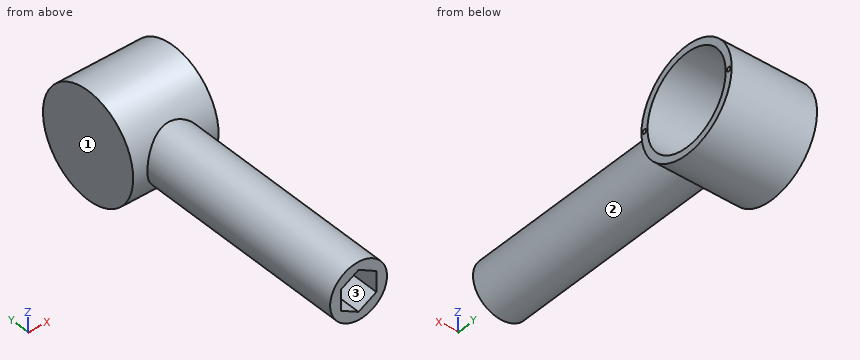
from build123d import *

# Parameters (mm, degrees)
SKETCH1_R                 = 20
BOSS_EXTRUDE1_DEPTH       = 25
BOSS_EXTRUDE2_START       = 100
SKETCH2_R                 = 20
BOSS_EXTRUDE2_DEPTH       = 100
BOSS_EXTRUDE4_START       = -100
SKETCH6_R                 = 20
BOSS_EXTRUDE4_DEPTH       = 100
SKETCH7_R                 = 25
CUT_EXTRUDE2_DEPTH        = 40
SKETCH8_R                 = 25
SKETCH8_R_2               = 22.5
BOSS_EXTRUDE7_DEPTH       = 40
SKETCH9_R                 = 25
BOSS_EXTRUDE8_DEPTH       = 2
BOSS_EXTRUDE10_DEPTH      = 38
CUT_EXTRUDE3_DEPTH        = 25
SKETCH12_R                = 25
CUT_EXTRUDE4_DEPTH        = 75
BOSS_EXTRUDE11_START      = 50
SKETCH14_R                = 20
BOSS_EXTRUDE11_DEPTH      = 50
BOSS_EXTRUDE12_DEPTH      = 10
BOSS_EXTRUDE12_DEPTH_BACK = 50
SKETCH13_R                = 37.5
SKETCH17_R                = 32.5
CUT_EXTRUDE5_DEPTH        = 50
BOSS_EXTRUDE13_START      = 2
SKETCH18_R                = 37.5
SKETCH18_R_2              = 32.5
BOSS_EXTRUDE13_DEPTH      = 2
SKETCH21_R                = 37.5
SKETCH21_R_2              = 32.5
CUT_EXTRUDE6_DEPTH        = 2
SKETCH22_R                = 1.5
CUT_EXTRUDE7_DEPTH        = 10
BOSS_EXTRUDE14_START      = 5
SKETCH27_R                = 32.5
BOSS_EXTRUDE14_DEPTH      = 5


with BuildPart() as part:
    # Sketch1 → Boss-Extrude1 (new body)
    with BuildSketch(Plane(origin=(0, 0, 0), x_dir=(1, 0, 0), z_dir=(0, 1, 0))):
        with Locations(Location((0, 0, 0), (0, 0, 270))):
            Circle(SKETCH1_R)
        Polygon((14.43375673, 0), (7.216878365, 12.5), (-7.216878365, 12.5), (-14.43375673, 0), (-7.216878365, -12.5), (7.216878365, -12.5), align=None, mode=Mode.SUBTRACT)
    extrude(amount=BOSS_EXTRUDE1_DEPTH)

    # Sketch2 → Boss-Extrude2 (add)
    with BuildSketch(Plane.XZ.offset(BOSS_EXTRUDE2_START)):
        with Locations(Location((0, 0, 0), (0, 0, 270))):
            Circle(SKETCH2_R)
    extrude(amount=-BOSS_EXTRUDE2_DEPTH)

    # Sketch6 → Boss-Extrude4 (add)
    with BuildSketch(Plane(origin=(0, 25, 0), x_dir=(1, 0, 0), z_dir=(0, 1, 0)).offset(BOSS_EXTRUDE4_START)):
        with Locations(Location((0, 0, 0), (0, 0, 90))):
            Circle(SKETCH6_R)
    extrude(amount=BOSS_EXTRUDE4_DEPTH)

    # Sketch7 → Cut-Extrude2 (cut)
    with BuildSketch(Plane(origin=(20, 0, 0), x_dir=(0, 0, -1), z_dir=(1, 0, 0))):
        with Locations((0, 39.286563349)):
            Circle(SKETCH7_R)
    extrude(amount=-CUT_EXTRUDE2_DEPTH, mode=Mode.SUBTRACT)

    # Sketch8 → Boss-Extrude7 (add)
    with BuildSketch(Plane(origin=(20, 0, 0), x_dir=(0, 0, -1), z_dir=(1, 0, 0))):
        with Locations((0, 39.252781264)):
            Circle(SKETCH8_R)
        with Locations((0, 39.252781264)):
            Circle(SKETCH8_R_2, mode=Mode.SUBTRACT)
    extrude(amount=-BOSS_EXTRUDE7_DEPTH)

    # Sketch9 → Boss-Extrude8 (add)
    with BuildSketch(Plane(origin=(20, 0, 0), x_dir=(0, 0, -1), z_dir=(1, 0, 0))):
        with Locations((0, 39.252781264)):
            Circle(SKETCH9_R)
    extrude(amount=-BOSS_EXTRUDE8_DEPTH)

    # Sketch10 → Boss-Extrude10 (add)
    with BuildSketch(Plane.ZY.offset(-18)):
        with BuildLine():
            Line((-15.081099266, 22.555163323), (15.081099266, 22.555163323))
            ThreePointArc((15.081099266, 22.555163323), (0, 16.752781264), (-15.081099266, 22.555163323))
        make_face()
    extrude(amount=BOSS_EXTRUDE10_DEPTH)

    # Sketch11 → Cut-Extrude3 (cut)
    with BuildSketch(Plane.XZ.offset(100)):
        Polygon((12.5, 7.216878365), (0, 14.43375673), (0, 0), (12.5, 0), align=None)
        Polygon((0, 0), (0, 14.43375673), (-12.5, 7.216878365), (-12.5, -7.216878365), (0, -14.43375673), (12.5, -7.216878365), (12.5, 0), align=None)
    extrude(amount=-CUT_EXTRUDE3_DEPTH, mode=Mode.SUBTRACT)

    # Sketch12 → Cut-Extrude4 (cut)
    with BuildSketch(Plane(origin=(20, 0, 0), x_dir=(0, 0, -1), z_dir=(1, 0, 0))):
        with Locations((0, 39.252781264)):
            Circle(SKETCH12_R)
    extrude(amount=-CUT_EXTRUDE4_DEPTH, mode=Mode.SUBTRACT)

    # Sketch14 → Boss-Extrude11 (add)
    with BuildSketch(Plane.XZ.offset(100).offset(BOSS_EXTRUDE11_START)):
        with Locations(Location((0, 0, 0), (0, 0, 270))):
            Circle(SKETCH14_R)
        Polygon((0, -14.43375673), (12.5, -7.216878365), (12.5, 7.216878365), (0, 14.43375673), (-12.5, 7.216878365), (-12.5, -7.216878365), align=None, mode=Mode.SUBTRACT)
    extrude(amount=-BOSS_EXTRUDE11_DEPTH)

    # Sketch13 → Boss-Extrude12 (add, two sides: drawn at the far end of the back side and taken through both)
    with BuildSketch(Plane(origin=(20, 0, 0), x_dir=(0, 0, -1), z_dir=(1, 0, 0)).offset(-BOSS_EXTRUDE12_DEPTH_BACK)):
        with Locations((0, 39.33472939)):
            Circle(SKETCH13_R)
    extrude(amount=BOSS_EXTRUDE12_DEPTH + BOSS_EXTRUDE12_DEPTH_BACK)

    # Sketch17 → Cut-Extrude5 (cut)
    with BuildSketch(Plane(origin=(30, 0, 0), x_dir=(0, 0, -1), z_dir=(1, 0, 0))):
        with Locations((0, 39.33472939)):
            Circle(SKETCH17_R)
    extrude(amount=-CUT_EXTRUDE5_DEPTH, mode=Mode.SUBTRACT)

    # Sketch18 → Boss-Extrude13 (add)
    with BuildSketch(Plane(origin=(30, 0, 0), x_dir=(0, 0, -1), z_dir=(1, 0, 0)).offset(BOSS_EXTRUDE13_START)):
        with Locations((0, 39.33472939)):
            Circle(SKETCH18_R)
        with Locations((0, 39.33472939)):
            Circle(SKETCH18_R_2, mode=Mode.SUBTRACT)
    extrude(amount=-BOSS_EXTRUDE13_DEPTH)

    # Sketch21 → Cut-Extrude6 (cut)
    with BuildSketch(Plane(origin=(32, 0, 0), x_dir=(0, 0, -1), z_dir=(1, 0, 0))):
        with Locations((0, 39.33472939)):
            Circle(SKETCH21_R)
        with Locations((0, 39.33472939)):
            Circle(SKETCH21_R_2, mode=Mode.SUBTRACT)
    extrude(amount=-CUT_EXTRUDE6_DEPTH, mode=Mode.SUBTRACT)

    # Sketch22 → Cut-Extrude7 (cut)
    with BuildSketch(Plane(origin=(30, 0, 0), x_dir=(0, 0, -1), z_dir=(1, 0, 0))):
        with Locations((0, 74.33472939)):
            Circle(SKETCH22_R)
        with Locations((0, 4.33472939)):
            Circle(SKETCH22_R)
    extrude(amount=-CUT_EXTRUDE7_DEPTH, mode=Mode.SUBTRACT)

    # Sketch27 → Boss-Extrude14 (add)
    with BuildSketch(Plane(origin=(-20, 0, 0), x_dir=(0, 0, -1), z_dir=(1, 0, 0)).offset(BOSS_EXTRUDE14_START)):
        with Locations((0, 39.33472939)):
            Circle(SKETCH27_R)
    extrude(amount=-BOSS_EXTRUDE14_DEPTH)


solid = part.part
Can you work these out from the model? Positions are in its coordinate system, mm. Face numbers are marked on the shaded views. Give positions to 0.01 mm unless a question says otherwise; leave off trailing zeros. Loops run counter-clockwise (first coordinate to the right, second up) from the corner with the lowest first, then second, coordinate; pieces in that order, holes last. Notation, with made-up numbers: M -6.5,-39 L 21.5,-39 A4 cw 21.5,-33 Z; hole C 16.5,-30.5 d10. An arc over 180 degrees is marked long. One line per item, written item: value. Start each with the question number.
1) If we section it at D-D, the plane y = -3.5: Write out the boundary of the cut face in (x, z).
2) If we section it at B-B, the plane x = 7: Write out the boundary of the cut face in (y, z) (3 decimals).
3) If we section it at C-C, the plane z = 26: Write out the boundary of the cut face in (x, y), and give its area (3 significant figures).
4) If I drill on line 1 (Y direction, x = 25.25, z = 0); line 2 (Y direction, x = -11, z = -0.5); line 3 (Z direction, x = 1, y = -67), over which ranges is the centre line in solid material (lowest first)? Write a range as [from, to].
5) Thinking about a two-plate mould opening in X: for the marked faces 1, 2 and 3, which applies, +X half, -X half, draft (parallel to the pull), parting line (faces both ways), or undercut?
6) I'm going to push flat-ended pins straight in: pin 1 (2.5 mm diameter, centred on y = 74.33, z = 0, fed in from +X); pin 2 (2 mm diameter, centred on x = -18.5, z = 25.5, fed in from +Y); pin 3 (11.5 mm diameter, centred on y = -123, z = -1, fed in from -X). Where does each tip first touch, or does it pass through?
7) If we section it at A-A, the plane y = -77: Write out the boundary of the cut face in (x, z).
Completed:
1. outline: C 0,0 d40
2. outline: M -150,-18.735 L 6.85,-18.735 A37.5 ccw long 6.85,18.735 L -150,18.735 L -150,10.392 L -75,10.392 L -75,-10.392 L -150,-10.392 Z; hole C 39.335,0 d65
3. outline: M -30,12.31 L 30,12.31 L 30,19.83 L -15,19.83 L -15,58.83 L 30,58.83 L 30,66.36 L -30,66.36 Z
3. area: 1,490 mm^2
4. line 1: y = [1.83, 2.83], [5.83, 6.83], [71.83, 72.83], [75.83, 76.83]
4. line 2: y = [-75, 6.84], [71.83, 76.83]
4. line 3: z = [-19.97, 19.97]
5. face 1: -X half
5. face 2: parting line
5. face 3: undercut
6. pin 1: stops at x = 20
6. pin 2: stops at y = 67.72
6. pin 3: stops at x = -20
7. outline: C 0,0 d40; hole M -12.5,-7.22 L 0,-14.43 L 12.5,-7.22 L 12.5,7.22 L 0,14.43 L -12.5,7.22 Z
